Verification items for the finished model (mm, model axes). A direction names the side the tool comes from. Coordinates: 2 decimals unless noted, no trailing zeros. Order: outer loops, then holes, each group sorted by start corner. A loop starts at its lowest first (then second) coordinate and runs counter-clockwise, first axis right, second up. Notation, with made-up numbers: M 74,-14 L 97,-14 A23 cw 97,24 Z; hole C 87,36 d8. An arc over 180 degrees is marked long. Write item = value, one per line.
```python
from build123d import *

# Parameters (mm, degrees)
CYLINDER009_R     = 2.65
CYLINDER009_DEPTH = 30
CYLINDER008_R     = 4
CYLINDER008_DEPTH = 3.2
CYLINDER010_R     = 1.375
CYLINDER010_DEPTH = 10
CYLINDER011_R     = 2.6
CYLINDER011_DEPTH = 2.1
ARRAY002_X_COUNT  = 2
ARRAY002_X_PITCH  = 15
CYLINDER007_R     = 37.7
CYLINDER007_DEPTH = 63
CYLINDER013_R     = 42.7
CYLINDER013_DEPTH = 45
CYLINDER012_R     = 49.7
CYLINDER012_DEPTH = 32.5
SKETCH_R          = 2.2
POCKET_DEPTH      = 5
SKETCH001_R       = 4.4
SKETCH001_R_2     = 4
POCKET001_DEPTH   = 2
POCKET006_DEPTH   = 25
PAD002_DEPTH      = 5
SKETCH018_W       = 2
SKETCH018_H       = 4.5
POCKET016_DEPTH   = 5


with BuildPart() as cylinder009:
    # Cylinder009 → Cylinder009 (new body)
    with BuildSketch(Plane.XY.offset(63)):
        Circle(CYLINDER009_R)
    extrude(amount=CYLINDER009_DEPTH)


with BuildPart() as cylinder008:
    # Cylinder008 → Cylinder008 (new body)
    with BuildSketch(Plane.XY.offset(64.8)):
        Circle(CYLINDER008_R)
    extrude(amount=CYLINDER008_DEPTH)


with BuildPart() as cylinder010:
    # Cylinder010 → Cylinder010 (new body)
    with BuildSketch(Plane.XY):
        Circle(CYLINDER010_R)
    extrude(amount=CYLINDER010_DEPTH)


with BuildPart() as fusion005:
    # Cylinder011 → Cylinder011 (new body)
    with BuildSketch(Plane.XY):
        Circle(CYLINDER011_R)
    extrude(amount=CYLINDER011_DEPTH)

    # Fusion004: union Cylinder010
    add(cylinder010.part)


with BuildPart() as fusion005_1:
    # Fusion004 placement: moved
    add(fusion005.part.moved(Location((0, 0, 63))))

    # Array002 X: Fusion005 ×2


with BuildPart() as fusion005_2:
    add(fusion005_1.part)
    with Locations(*[(i * ARRAY002_X_PITCH, 0, 0) for i in range(1, ARRAY002_X_COUNT)]):
        add(fusion005_1.part)


with BuildPart() as fusion005_3:
    # Array002 placement: moved
    add(fusion005_2.part.moved(Location((-7.5, 0, 0))))

    # Fusion005: union Cylinder009, Cylinder008
    add(cylinder009.part)
    add(cylinder008.part)


with BuildPart() as cylinder007:
    # Cylinder007 → Cylinder007 (new body)
    with BuildSketch(Plane.XY):
        Circle(CYLINDER007_R)
    extrude(amount=CYLINDER007_DEPTH)


with BuildPart() as fusion006:
    # Cylinder013 → Cylinder013 (new body)
    with BuildSketch(Plane.XY):
        Circle(CYLINDER013_R)
    extrude(amount=CYLINDER013_DEPTH)

    # Fusion006: union Cylinder007
    add(cylinder007.part)


with BuildPart() as obj1:
    # Cylinder012 → Cylinder012 (new body)
    with BuildSketch(Plane.XY.offset(35.5)):
        Circle(CYLINDER012_R)
    extrude(amount=CYLINDER012_DEPTH)

    # Cut008: cut Fusion006
    add(fusion006.part, mode=Mode.SUBTRACT)

    # Cut009: cut Fusion005
    add(fusion005_3.part, mode=Mode.SUBTRACT)

    # Sketch (on Face3 of Cut009) → Pocket (cut)
    with BuildSketch(Plane.XY.offset(68)):
        with Locations((0, 25)):
            Circle(SKETCH_R)
        with Locations((25, 0)):
            Circle(SKETCH_R)
        with Locations((0, -25)):
            Circle(SKETCH_R)
        with Locations((-25, 0)):
            Circle(SKETCH_R)
    extrude(amount=-POCKET_DEPTH, mode=Mode.SUBTRACT)

    # Sketch001 (on Face13 of Pocket) → Pocket001 (cut)
    with BuildSketch(Plane(origin=(0, 0, 63), x_dir=(1, 0, 0), z_dir=(0, 0, -1))):
        with Locations((-25, 0)):
            Circle(SKETCH001_R)
        with Locations((0, 25)):
            Circle(SKETCH001_R_2)
        with Locations((25, 0)):
            Circle(SKETCH001_R_2)
        with Locations((0, -25)):
            Circle(SKETCH001_R_2)
    extrude(amount=-POCKET001_DEPTH, mode=Mode.SUBTRACT)

    # Sketch002 → Pocket006 (cut)
    with BuildSketch(Plane(origin=(0, 60, -1), x_dir=(1, 0, 0), z_dir=(0, -1, 0))):
        with BuildLine():
            ThreePointArc((3.4, 59.599979), (1.2e-05, 63), (-3.4, 59.600003))
            Line((-3.4, 59.600003), (-3.4, 0))
            Line((-3.4, 0), (3.4, 0))
            Line((3.4, 59.599979), (3.4, 0))
        make_face()
    extrude(amount=POCKET006_DEPTH, mode=Mode.SUBTRACT)

    # Sketch017 (on Face2 of Pocket006) → Pad002 (join)
    with BuildSketch(Plane(origin=(0, 0, 35.5), x_dir=(1, 0, 0), z_dir=(0, 0, -1))):
        with BuildLine():
            ThreePointArc((20.231067, 45.395694), (-0.005277, 49.699749), (-20.240706, 45.391396))
            Line((-7.40759, 82.752427), (-20.240706, 45.391396))
            ThreePointArc((7.358623, 82.756756), (-0.025675, 86.818946), (-7.40759, 82.752427))
            Line((7.358623, 82.756756), (20.231067, 45.395694))
        make_face()
    extrude(amount=-PAD002_DEPTH)

    # Sketch018 (on Face22 of Pad002) → Pocket016 (cut)
    with BuildSketch(Plane(origin=(0, 0, 35.5), x_dir=(1, 0, 0), z_dir=(0, 0, -1))):
        with Locations((0, 67.25)):
            Rectangle(SKETCH018_W, SKETCH018_H)
    extrude(amount=-POCKET016_DEPTH, mode=Mode.SUBTRACT)


solid = obj1.part
```
Item 1: Sectioned sample at B-B, the plane y = -25. Enter the section's corners in (x, z), then the cut area to 3 significant figures.
Report:
outline = M -42.95,35.5 L -34.62,35.5 L -34.62,45 L -28.22,45 L -28.22,63 L -4,63 L -4,65 L -2.2,65 L -2.2,68 L -42.95,68 Z; M 2.2,65 L 4,65 L 4,63 L 28.22,63 L 28.22,45 L 34.62,45 L 34.62,35.5 L 42.95,35.5 L 42.95,68 L 2.2,68 Z
area = 1,090 mm^2
Item 2: Gauge pin test, flat ends, axial feed: pin 1 (9 mm diameter, centred on x = 26, y = -2, fed in from -Z); pin 2 (6 mm diameter, centred on y = 36, z = 45, fed in from -X); pin 3 (1.3 mm diameter, centred on y = -68, z = 37, fed in from +X); pin 4 (2 mm diameter, centred on x = 7.5, y = 0, fed in from +Z) (3 decimals). Record the tip position at first contact, or that the pin passes through.
Report:
pin_1 = 63
pin_2 = -37.16
pin_3 = 12.67
pin_4 = through
Item 3: Sectioned sample at A-A, the plane x = -25. Enter the section's corners in (y, z), then the cut area to 3 significant figures.
Report:
outline = M -42.95,35.5 L -34.62,35.5 L -34.62,45 L -28.22,45 L -28.22,63 L -4.4,63 L -4.4,65 L -2.2,65 L -2.2,68 L -42.95,68 Z; M 2.2,65 L 4.4,65 L 4.4,63 L 28.22,63 L 28.22,45 L 34.62,45 L 34.62,35.5 L 42.95,35.5 L 42.95,68 L 2.2,68 Z
area = 1,090 mm^2
Item 4: Sectioned sample at C-C, the plane x = 35. Enter the section's corners in (y, z).
Report:
outline = M -35.29,35.5 L -24.46,35.5 L -24.46,45 L -14.01,45 L -14.01,63 L 14.01,63 L 14.01,45 L 24.46,45 L 24.46,35.5 L 35.29,35.5 L 35.29,68 L -35.29,68 Z
Item 5: Sectioned sample at D-D, the plane z = 50. Enter the section's corners in (x, y), then the cut area to 3 significant figures.
Report:
outline = M -3.4,37.55 L -3.4,49.58 A49.7 ccw long 3.4,49.58 L 3.4,37.55 A37.7 cw long Z
area = 3,210 mm^2
Item 6: Scan lines: L1, parallel to Y at x = 0, z = 63.95; L2, parallel to Y at x = 0, z = 66.9; L3, parallel to Z at x = 27.5, y = 18. Record each from-to range of solid material in increasing order. Write a range as from..to.
Report:
L1 = -49.7..-29, -21..-2.65, 2.65..21, 29..49.7
L2 = -49.7..-27.2, -22.8..-4, 4..22.8, 27.2..49.7
L3 = 63..68
Item 7: Tool access check on faces 1 (the cylindrical face through (-8.173, -36.804, 53.874)), 2 (the cylindrical face through (0, 44, 62)), 3 (the flat face through (3, -1, 64.8)). Record the directions out of +Z, -Z, +X, -X, +Y, -Y that give a thin tool (end or side, any length) a straight path to the whole face; none if there is none.
Report:
face_1 = -Z
face_2 = -Z, +Y
face_3 = +Z
